Could you check a few things on this model? Use its own coordinates, in mm. A direction names the side the tool comes from. Give positions to 0.01 mm unless a question says otherwise; leave off trailing zeros. Put each result on its own line as item: value.
Autodesk Fusion 360 part; units mm, degrees
sketch "Sketch1" plane through (0, 0, 0) normal (0, 0, 1) x (1, 0, 0)
  line L0 (0, 0) -> (254, 0)
  line L1 (254, 0) -> (254, 254)
  line L2 (254, 254) -> (0, 254)
  line L3 (0, 254) -> (0, 0)
  line L4 (0, 127) -> (254, 127) construction
  line L5 (251, 200) -> (254, 200)
  line L6 (254, 204) -> (251, 204)
  arc A0 (251, 204) -> (251, 200) centre (251, 202) ccw
  line L7 (251, 202) -> (275, 202) construction
  line L8 (251, 50) -> (254, 50)
  line L9 (254, 54) -> (251, 54)
  arc A1 (251, 54) -> (251, 50) centre (251, 52) ccw
  line L10 (251, 52) -> (254, 52) construction
  line L11 (3, 204) -> (0, 204)
  line L12 (0, 200) -> (3, 200)
  arc A2 (3, 200) -> (3, 204) centre (3, 202) ccw
  line L13 (3, 202) -> (0, 202) construction
  line L14 (254, 205.25) -> (251, 205.25)
  arc A3 (251, 205.25) -> (251, 198.75) centre (251, 202) ccw
  line L15 (251, 198.75) -> (254, 198.75)
  line L16 (254, 55.25) -> (251, 55.25)
  arc A4 (251, 55.25) -> (251, 48.75) centre (251, 52) ccw
  line L17 (251, 48.75) -> (254, 48.75)
  line L18 (0, 198.75) -> (3, 198.75)
  arc A5 (3, 198.75) -> (3, 205.25) centre (3, 202) ccw
  line L19 (3, 205.25) -> (0, 205.25)
  line L20 (3, 54) -> (0, 54)
  line L21 (0, 50) -> (3, 50)
  arc A6 (3, 50) -> (3, 54) centre (3, 52) ccw
  line L22 (3, 52) -> (0, 52) construction
  line L23 (0, 48.75) -> (3, 48.75)
  arc A7 (3, 48.75) -> (3, 55.25) centre (3, 52) ccw
  line L24 (3, 55.25) -> (0, 55.25)
  point P0 (251, 202)
  point P1 (251, 52)
  point P2 (3, 52)
  point P3 (3, 202)
  dimension "d3" = 254
  dimension "d4" = 254
  dimension "d8" = 3
  dimension "d9" = 3
  dimension "d10" = 75
  dimension "d11" = 75
  dimension "d12" = 2
  dimension "d13" = 2
  dimension "d15" = 3
  dimension "d16" = 75
  dimension "d19" = 2
  dimension "d20" = 1.25
  dimension "d21" = 1.25
  dimension "d22" = 1.25
  dimension "d94" = 127
  dimension "d95" = 3
  dimension "d96" = 2
  dimension "d97" = 75
  dimension "d98" = 1.25
extrude "Extrude2" add sketch "Sketch1" along normal blind 4.95 contours L0 L1 L2 L3 L14 A3 L15 L16 A4 L17 L18 A5 L19 L23 A7 L24
extrude "Extrude3" add sketch "Sketch1" against normal blind 3 contours L0 L1 L2 L3 L14 A3 L15 L16 A4 L17 L18 A5 L19 L23 A7 L24 | L3 L20 L21 A6 L23 A7 L24 | L1 L8 L9 A1 L16 A4 L17 | L3 L11 L12 A2 L18 A5 L19 | L1 L5 L6 A0 L14 A3 L15
chamfer "Chamfer6" distance 0.5 angle 45 16 edges at (0, 205.25, 2.475) (0, 198.75, 2.475) (0, 204, -1.5) (0, 200, -1.5) (0, 55.25, 2.475) (0, 48.75, 2.475) (0, 50, -1.5) (0, 54, -1.5) (254, 48.75, 2.475) (254, 55.25, 2.475) (254, 54, -1.5) (254, 50, -1.5) (254, 205.25, 2.475) (254, 198.75, 2.475) (254, 200, -1.5) (254, 204, -1.5)
equation "x_bed_size = 10 in"
equation "y_bed_size = 10 in"
equation "d3 = x_bed_size"
equation "d4 = y_bed_size"
equation "d8 = d9"
equation "d10 = ( 150 / 2 ) * 1 mm"
equation "d11 = d10"
equation "d12 = d13"
equation "d15 = d9"
equation "d16 = d10"
equation "d19 = d13"
equation "d21 = d20"
equation "d22 = d20"
equation "d23 = 7.95 mm - 3 mm"
equation "d94 = y_bed_size / 2"
equation "d95 = d15"
equation "d96 = d19"
equation "d97 = d16"
1. For faces 1 (the face through (0, 230, 1)), 2 (the face through (5, 201, 0)), which set-ups out of +Z, -Z, +X, -X, +Y, -Y let a thin tool reach every point of the face, with its end or its side?
Recorded:
face 1: +Z, -Z, -X, +Y, -Y
face 2: +Z, -X
2. I'm going to push flat-ended pins straight in: pin 1 (0.8 mm diameter, centred on x = 252, z = -2, fed in from -Y); pin 2 (3 mm diameter, centred on x = 251.5, y = 201, fed in from +Z); pin 3 (1.9 mm diameter, centred on x = 2, y = 52, fed in from +Z). Where does each tip first touch, or does it pass through?
Recorded:
pin 1: stops at y = 0
pin 2: stops at z = 0
pin 3: passes through
3. Thinking about a two-plate mould opening in Y: for faces 3 (the face through (254, 229, 1)), 4 (the face through (129, 254, 1)), 5 (the face through (249, 201, 0)), 6 (the face through (249, 51, 0)), which applies, pulls with the +Y half, pulls with the -Y half, needs draft (parallel to the pull), parting line crosses it, or undercut?
Recorded:
face 3: needs draft
face 4: pulls with the +Y half
face 5: undercut
face 6: undercut
